from build123d import *

# Parameters (mm, degrees)
SKETCH_1_R          = 14
SKETCH_1_R_2        = 1.475
SKETCH_1_R_3        = 4.95
EXTRUDE_1_DEPTH     = 2.2
SKETCH_1_3_R        = 4.95
SKETCH_1_3_R_2      = 1.5
EXTRUDE_2_DEPTH     = 5
SKETCH_2_R          = 2.925
CUT_EXTRUDE_1_DEPTH = 3.2
CUT_EXTRUDE_2_DEPTH = 1


with BuildPart() as part:
    # Sketch 1 → Extrude 1 (new body)
    with BuildSketch(Plane(origin=(0, 0, 0), x_dir=(1, 0, 0), z_dir=(0, 1, 0))):
        with Locations(Location((0, 0, 0), (0, 0, 270))):
            Circle(SKETCH_1_R)
        with Locations(Location((7.075, -7.075, 0), (0, 0, 270))):
            Circle(SKETCH_1_R_2, mode=Mode.SUBTRACT)
        with Locations(Location((7.075, 7.075, 0), (0, 0, 270))):
            Circle(SKETCH_1_R_2, mode=Mode.SUBTRACT)
        with Locations(Location((0, 0, 0), (0, 0, 270))):
            Circle(SKETCH_1_R_3, mode=Mode.SUBTRACT)
        with Locations(Location((-7.075, 7.075, 0), (0, 0, 270))):
            Circle(SKETCH_1_R_2, mode=Mode.SUBTRACT)
        with Locations(Location((-7.075, -7.075, 0), (0, 0, 270))):
            Circle(SKETCH_1_R_2, mode=Mode.SUBTRACT)
    extrude(amount=EXTRUDE_1_DEPTH)

    # Sketch 1_3 → Extrude 2 (add)
    with BuildSketch(Plane(origin=(0, 0, 0), x_dir=(1, 0, 0), z_dir=(0, 1, 0))):
        with Locations(Location((0, 0, 0), (0, 0, 270))):
            Circle(SKETCH_1_3_R)
        with Locations(Location((0, 0, 0), (0, 0, 270))):
            Circle(SKETCH_1_3_R_2, mode=Mode.SUBTRACT)
    extrude(amount=EXTRUDE_2_DEPTH)

    # Sketch 2 → Cut-Extrude 1 (cut)
    with BuildSketch(Plane(origin=(0, 5, 0), x_dir=(1, 0, 0), z_dir=(0, 1, 0))):
        with Locations(Location((0, 0, 0), (0, 0, 270))):
            Circle(SKETCH_2_R)
    extrude(amount=-CUT_EXTRUDE_1_DEPTH, mode=Mode.SUBTRACT)

    # Sketch 3 → Cut-Extrude 2 (cut)
    with BuildSketch(Plane.XZ):
        Polygon((0.707106781, 0.707106781), (-0.707106781, -0.707106781), (-2.828427125, 1.414213562), (-1.414213562, 2.828427125), align=None)
    extrude(amount=-CUT_EXTRUDE_2_DEPTH, mode=Mode.SUBTRACT)


solid = part.part
For this review, take the finished solid that the model builds, in its own axes (mm). A direction names the side the tool comes from. Give positions to 0.01 mm unless a question says otherwise; leave off trailing zeros. Loops run counter-clockwise (first coordinate to the right, second up) from the corner with the lowest first, then second, coordinate; pieces in that order, holes last. Notation, with made-up numbers: M -31,-21 L 17,-21 A11 cw 17,-13 Z; hole C -1,-20.5 d5. An arc over 180 degrees is marked long. Answer as a JSON object with one key per item and string values. Group by question number.
Q1. Add section D-D on y = 3.85. Give the boundary of the cut face in (x, z) (3 decimals).
Q2. Tool access review of faces 1 (the flat face through (-2.154, 0.493, 0.74)), 2 (the flat face through (-6, 2.2, 0)), 3 (the cylindrical face through (8.072, 1.085, -8.162)): name each direction out of +Z, -Z, +X, -X, +Y, -Y from which nothing blocks a thin tool from reaching the whole face with its end or side.
Q3. Mouldability with a two-part tool opening along Z and no side actions: class faces 4 (the flat face through (-3.2, 5, -0.1)), 5 (the cylindrical face through (1.49, 3.58, 4.72)), 6 (the cylindrical face through (1.01, 0.89, -1.11)), 7 (the flat face through (-1.3, 1.8, 1.3)) as +Z half, -Z half, draft (parallel to the pull), parting line (faces both ways), or undercut.
Q4. For probe 1 along X at (y, z) = (2.65, 0) (3 decimals); probe 2 along Y at (x, z) = (9.25, -3.25); probe 3 along X at (y, z) = (0.7, -0.5), list the stretches that pass through material, from the lowest coordinate up. Write a range as [from, to].
Q5. Add section C-C on x = 0.5. Give the boundary of the cut face in (y, z), and give its area (3 significant figures).
Q6. Add section B-B on x = 6. Give the boundary of the cut face in (y, z), and give its area (3 significant figures).
Q7. Add section A-A on z = 6.25. Give the boundary of the cut face in (x, y).
Q8. Insertion check: P1, Ø1.8, axis at x = 7.075, z = -7.075, coming from the +Y side; P2, Ø1.8, axis at x = -0.5, z = 1, coming from the +Y side; P3, Ø3, axis at x = -5.5, z = 5, coming from the +Y side; P4, Ø1.5, axis at x = -5, y = 4, coming from the +Z side. Each pin has a flat end and moves straight along its axis. Give the tip position at first contact, or say it passes through.
Checked values:
{
 "1": {"outline": "C 0,0 d9.9; hole C 0,0 d5.85"},
 "2": {"face 1": "-Y", "face 2": "+Y", "face 3": "+Y, -Y"},
 "3": {"face 4": "draft", "face 5": "parting line", "face 6": "undercut", "face 7": "undercut"},
 "4": {"probe 1": "[-4.95, -2.925], [2.925, 4.95]", "probe 2": "[0, 2.2]", "probe 3": "[-13.99, -1.41], [1.41, 13.99]"},
 "5": {"outline": "M 0,-13.99 L 2.2,-13.99 L 2.2,-4.92 L 5,-4.92 L 5,-2.88 L 1.8,-2.88 L 1.8,-1.41 L 0,-1.41 Z; M 0,1.41 L 1.8,1.41 L 1.8,2.88 L 5,2.88 L 5,4.92 L 2.2,4.92 L 2.2,13.99 L 0,13.99 Z", "area": "65.6 mm²"},
 "6": {"outline": "M 0,-12.65 L 2.2,-12.65 L 2.2,-8.08 L 0,-8.08 Z; M 0,-6.07 L 2.2,-6.07 L 2.2,6.07 L 0,6.07 Z; M 0,8.08 L 2.2,8.08 L 2.2,12.65 L 0,12.65 Z", "area": "46.8 mm²"},
 "7": {"outline": "M -12.53,0 L -8.3,0 L -8.3,2.2 L -12.53,2.2 Z; M -5.85,0 L 5.85,0 L 5.85,2.2 L -5.85,2.2 Z; M 8.3,0 L 12.53,0 L 12.53,2.2 L 8.3,2.2 Z"},
 "8": {"P1": "through", "P2": "y = 1.8", "P3": "y = 2.2", "P4": "z = 2.54"}
}
